Verification items for the finished model (mm, model axes). A direction names the side the tool comes from. Round coordinates to 2 decimals unless told otherwise and drop trailing zeros. Loops run counter-clockwise (first coordinate to the right, second up) from the corner with the lowest first, then second, coordinate; pieces in that order, holes last. Notation, with made-up numbers: (-35.75, 40.5) - (-19.75, 40.5) arc R25 ccw to (-19.75, 64.5) - close; hole circle Ø8 at (35, 31.25). An arc over 180 degrees is marked (long way). Use CSV: the item, a comma, the result in double quotes.
Autodesk Fusion 360 part; units mm, degrees
sketch "machine arm" plane through (0, 0, 0) normal (0, 0, 1) x (1, 0, 0)
  line L0 (-50, -25) -> (50, -25)
  line L1 (50, -25) -> (50, 25)
  line L2 (50, 25) -> (-50, 25)
  line L3 (-50, 25) -> (-50, -25)
  line L4 (-50, -25) -> (50, 25) construction
  line L5 (50, -25) -> (-50, 25) construction
  dimension "d1" = 100
  dimension "d2" = 50
extrude "Extrude1" add sketch "machine arm" along normal blind 10
sketch "socket" plane through (0, 0, 0) normal (0, 0, -1) x (1, 0, 0)
  line L0 (-50, 25) -> (-50, -25)
  line L1 (-50, -25) -> (50, -25)
  line L2 (50, -25) -> (50, 25)
  line L3 (50, 25) -> (-50, 25)
  line L4 (47.5, 10) -> (32.5, 10)
  line L5 (32.5, 10) -> (32.5, -10)
  line L6 (32.5, -10) -> (47.5, -10)
  line L7 (47.5, -10) -> (47.5, 10)
  line L8 (47.5, 10) -> (32.5, -10) construction
  line L9 (32.5, 10) -> (47.5, -10) construction
  point P0 (40, 0)
  dimension "d5" = 15
  dimension "d6" = 20
extrude "Extrude2" cut sketch "socket" against normal blind 5 contours L4 L5 L6 L7
sketch "Sketch3" plane through (0, 0, 10) normal (0, 0, 1) x (-1, 0, 0)
  line L0 (50, -25) -> (50, 25)
  line L1 (50, 25) -> (-50, 25)
  line L2 (-50, 25) -> (-50, -25)
  line L3 (-50, -25) -> (50, -25)
  line L4 (25, -20) -> (45, -20)
  line L5 (45, -20) -> (45, 20)
  line L6 (45, 20) -> (25, 20)
  line L7 (25, 20) -> (25, -20)
  point P0 (25, -20)
extrude "Extrude3" add sketch "Sketch3" along normal blind 5 contours L4 L5 L6 L7
1) Mould release check, pull along X, two halves, no side actions. Record for faces 1 (the face through (40, 10, 2)), 2 (the face through (50, 0, 5)), 3 (the face through (1, 25, 5)): +X half, -X half, draft (parallel to the pull), parting line (faces both ways), or undercut.
Returned:
face 1,"undercut"
face 2,"+X half"
face 3,"draft"
2) Cross-section at B-B, the plane x = 43. Record the cut outline in (y, z), then the cut area to 3 significant figures.
Returned:
outline,"(-25, 0) - (-10, 0) - (-10, 5) - (10, 5) - (10, 0) - (25, 0) - (25, 10) - (-25, 10) - close"
area,"400 mm²"
3) Access from +Z, -Z, +X, -X, +Y, -Y to the whole of each face (thin tool, end or side, straight path). Record for faces 4 (the face through (-25, 0, 12)), 5 (the face through (-45, 0, 12)), 6 (the face through (-35, -20, 12)), 7 (the face through (32.5, 0, 2)).
Returned:
face 4,"+Z, +X, +Y, -Y"
face 5,"+Z, -X, +Y, -Y"
face 6,"+Z, +X, -X, -Y"
face 7,"-Z"
4) Gauge pin test, flat ends, axial feed: pin 1 Ø12 at (x, y) = (26, 7) entering from -Z; pin 2 Ø1 at (y, z) = (-17.5, 11) entering from -X; pin 3 Ø2 at (y, z) = (14.5, 11.5) entering from +X; pin 4 Ø4 at (x, z) = (-31, 13.5) entering from -Y. Record the tip position at first contact, or that the pin passes through.
Returned:
pin 1,"stops at z = 0"
pin 2,"stops at x = -45"
pin 3,"stops at x = -25"
pin 4,"stops at y = -20"
5) Thickness scan on probe 1 along Z at (x, y) = (3.5, -11); probe 2 along X at (y, z) = (19, 14); probe 3 along Z at (x, y) = (44, 6). Record the ranges inside material, lowest first. Write a range as [from, to].
Returned:
probe 1,"z = [0, 10]"
probe 2,"x = [-45, -25]"
probe 3,"z = [5, 10]"
6) Cross-section at A-A, the plane z = 1.5. Record the cut outline in (x, y), then the cut area to 3 significant figures.
Returned:
outline,"(-50, -25) - (50, -25) - (50, 25) - (-50, 25) - close; hole (32.5, -10) - (47.5, -10) - (47.5, 10) - (32.5, 10) - close"
area,"4,700 mm²"
7) Cross-section at D-D, the plane y = 15.5. Record the cut outline in (x, z).
Returned:
outline,"(-50, 0) - (50, 0) - (50, 10) - (-25, 10) - (-25, 15) - (-45, 15) - (-45, 10) - (-50, 10) - close"
8) Cross-section at C-C, the plane y = 2. Record the cut outline in (x, z), then the cut area to 4 significant figures.
Returned:
outline,"(-50, 0) - (32.5, 0) - (32.5, 5) - (47.5, 5) - (47.5, 0) - (50, 0) - (50, 10) - (-25, 10) - (-25, 15) - (-45, 15) - (-45, 10) - (-50, 10) - close"
area,"1,025 mm²"
